Can you work these out from the model? Positions are in its coordinate system, mm. Coordinates: 2 decimals unless noted, no trailing zeros. Order: outer loops, then holes, each group sorted by start corner. A loop starts at its lowest first (then second) coordinate and runs counter-clockwise, first axis right, second up. Notation, with made-up numbers: M 62,73.25 L 81,73.25 A15 ccw 81,78.25 Z; hole C 21.25,29.5 d7. An arc over 180 degrees is marked long. Answer as a JSON object with one key per item and string values.
from build123d import *

# Parameters (mm, degrees)
SKETCH_9_R      = 1.6
SKETCH_9_R_2    = 73.9
EXTRUDE_4_DEPTH = 5


with BuildPart() as part:
    # 草图9 → 凸台-拉伸4 (new body)
    with BuildSketch(Plane(origin=(0, 0, 0), x_dir=(1, 0, 0), z_dir=(0, 1, 0))):
        with BuildLine():
            ThreePointArc((136.437456541, -26.366693536), (126.517308136, 0), (136.437456541, 26.366693536))
            ThreePointArc((136.437456541, 26.366693536), (132.936074863, 132.936074863), (26.366693536, 136.437456541))
            ThreePointArc((26.366693536, 136.437456541), (0, 126.517308136), (-26.366693536, 136.437456541))
            ThreePointArc((-26.366693536, 136.437456541), (-132.936074863, 132.936074863), (-136.437456541, 26.366693536))
            ThreePointArc((-136.437456541, 26.366693536), (-126.517308136, 0), (-136.437456541, -26.366693536))
            ThreePointArc((-136.437456541, -26.366693536), (-132.936074863, -132.936074863), (-26.366693536, -136.437456541))
            ThreePointArc((-26.366693536, -136.437456541), (0, -126.517308136), (26.366693536, -136.437456541))
            ThreePointArc((26.366693536, -136.437456541), (132.936074863, -132.936074863), (136.437456541, -26.366693536))
        make_face()
        with Locations(Location((0, -80, 0), (0, 0, 270))):
            Circle(SKETCH_9_R, mode=Mode.SUBTRACT)
        with Locations(Location((-77.781745931, -77.781745931, 0), (0, 0, 270))):
            Circle(SKETCH_9_R_2, mode=Mode.SUBTRACT)
        with Locations(Location((77.781745931, -77.781745931, 0), (0, 0, 270))):
            Circle(SKETCH_9_R_2, mode=Mode.SUBTRACT)
        with Locations(Location((-90, 0, 0), (0, 0, 270))):
            Circle(SKETCH_9_R, mode=Mode.SUBTRACT)
        with Locations(Location((-70, 0, 0), (0, 0, 270))):
            Circle(SKETCH_9_R, mode=Mode.SUBTRACT)
        with Locations(Location((-77.781745931, 77.781745931, 0), (0, 0, 270))):
            Circle(SKETCH_9_R_2, mode=Mode.SUBTRACT)
        with Locations(Location((0, 80, 0), (0, 0, 270))):
            Circle(SKETCH_9_R, mode=Mode.SUBTRACT)
        with BuildLine():
            ThreePointArc((68.43730817, -0.343502905), (26.010818803, -19.439898991), (2.004358454, -59.29424888))
            ThreePointArc((2.004358454, -59.29424888), (-17.301800102, -22.556876962), (-52.137838272, 0))
            ThreePointArc((-52.137838272, 0), (-17.301800102, 22.556876962), (2.004358454, 59.29424888))
            ThreePointArc((2.004358454, 59.29424888), (26.010818803, 19.439898991), (68.43730817, 0.343502905))
            ThreePointArc((68.43730817, 0.343502905), (70.159278325, 1.592052265), (71.599770286, 0.027111489))
            ThreePointArc((71.599770286, 0.027111489), (71.775266864, 0.013357692), (71.950794036, 0))
            ThreePointArc((71.950794036, 0), (71.775266864, -0.013357692), (71.599770286, -0.027111489))
            ThreePointArc((71.599770286, -0.027111489), (70.159278325, -1.592052265), (68.43730817, -0.343502905))
        make_face(mode=Mode.SUBTRACT)
        with Locations(Location((77.781745931, 77.781745931, 0), (0, 0, 270))):
            Circle(SKETCH_9_R_2, mode=Mode.SUBTRACT)
        with Locations(Location((90, 0, 0), (0, 0, 270))):
            Circle(SKETCH_9_R, mode=Mode.SUBTRACT)
    extrude(amount=EXTRUDE_4_DEPTH)


solid = part.part
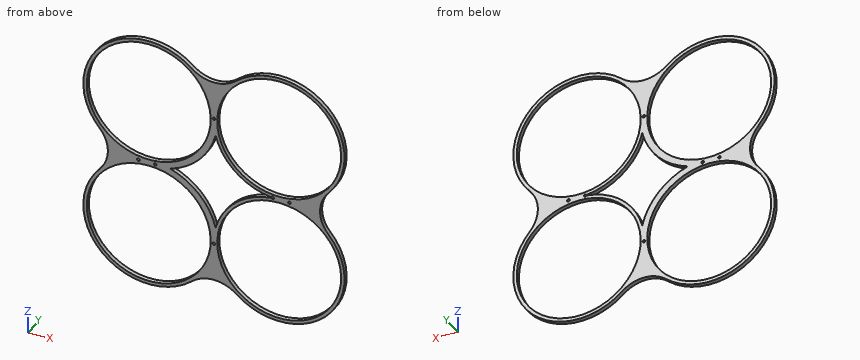
Item 1: I want a section at A-A, the plane z = -104. Write out the boundary of the cut face in (x, y), plus the area to 3 significant figures.
Answers follow:
{"outline": "M -151.24,0 L -146.87,0 L -146.87,5 L -151.24,5 Z; M -8.69,0 L 8.69,0 L 8.69,5 L -8.69,5 Z; M 146.87,0 L 151.24,0 L 151.24,5 L 146.87,5 Z", "area": "131 mm^2"}
Item 2: Please list where these lines run through material, in increasing order: line 1 (X direction, y = 3.7, z = 42.5); line 2 (X direction, y = 0.85, z = 143) (3 decimals); line 3 (Z direction, x = -44.5, y = 2.15).
Answers follow:
{"line 1": "x = -147.35 to -142.72, -12.85 to -3.87, 8.22 to 12.85, 142.72 to 147.35", "line 2": "x = -120.567 to -112.535, -43.028 to -34.996, 34.996 to 43.028, 112.535 to 120.567", "line 3": "z = -148.32 to -143.76, -11.8 to -2.95, 2.95 to 11.8, 143.76 to 148.32"}
Item 3: I want a section at C-C, the plane x = -84.5. Write out the boundary of the cut face in (y, z), plus the area to 3 significant figures.
Answers follow:
{"outline": "M 0,-155.49 L 5,-155.49 L 5,-151.38 L 0,-151.38 Z; M 0,-4.19 L 5,-4.19 L 5,4.19 L 0,4.19 Z; M 0,151.38 L 5,151.38 L 5,155.49 L 0,155.49 Z", "area": "83.0 mm^2"}
Item 4: I'm going to push flat-ended pins straight in: pin 1 (1 mm diameter, centred on y = 3, z = 90.5, fed in from +X); pin 2 (2 mm diameter, centred on x = 16.5, y = 0.5, fed in from -Z); pin 3 (1.5 mm diameter, centred on x = 84, y = 0.5, fed in from -Z). Where does each tip first touch, or does it pass through?
Answers follow:
{"pin 1": "stops at x = 154.82", "pin 2": "stops at z = -130.55", "pin 3": "stops at z = -155.59"}
Item 5: I want a section at D-D, the plane y = 2. Give the number of separate pieces and of enclosed holes in the cut face, plus the area to 3 significant figures.
Answers follow:
{"separate pieces": "1", "enclosed holes": "10", "area": "10,800 mm^2"}
Item 6: I want a section at B-B, the plane x = -40. Write out the boundary of the cut face in (y, z).
Answers follow:
{"outline": "M 0,-146.02 L 5,-146.02 L 5,-141.29 L 0,-141.29 Z; M 0,-14.27 L 5,-14.27 L 5,-5.12 L 0,-5.12 Z; M 0,5.12 L 5,5.12 L 5,14.27 L 0,14.27 Z; M 0,141.29 L 5,141.29 L 5,146.02 L 0,146.02 Z"}
